```python
from build123d import *

# Parameters (mm, degrees)
F_6_X_6_ANGLE_BAR_EXTRUSION_DEPTH = 63.5
EXTRUSION_FILLETS_R               = 6.35
F_10_CLEARANCE_HOLE_ROUTER_D      = 5.1054
SKETCH7_R                         = 13.49375
F_1_OD_BIT_ACCESS_HOLE_DEPTH      = 219.337526836
TAPPED_HOLE_FOR_10_32_HELICOIL1_D = 5.1054
MOUNTING_SLOTS_REACH              = 226.686


with BuildPart() as part:
    # Sketch1 → 6" x 6" angle bar extrusion (new, symmetric)
    with BuildSketch(Plane(origin=(0, 0, 0), x_dir=(0, 0, -1), z_dir=(1, 0, 0))):
        Polygon((0, 0), (0, 152.4), (-9.525, 152.4), (-9.525, 9.525), (-152.4, 9.525), (-152.4, 0), align=None)
    extrude(amount=F_6_X_6_ANGLE_BAR_EXTRUSION_DEPTH, both=True)

    # extrusion fillets
    extrusion_fillets_edges = [part.edges().sort_by_distance(p)[0] for p in [
        (0, 9.525, 152.4),
        (0, 9.525, 9.525),
        (0, 152.4, 9.525),
    ]]
    fillet(extrusion_fillets_edges, radius=EXTRUSION_FILLETS_R)

    # #10 Clearance Hole - router (through all)
    with Locations(Plane(origin=(0, 9.525, 0), x_dir=(1, 0, 0), z_dir=(0, 1, 0))):
        with Locations((-34.29, -25.4), (34.29, -101.6), (-34.29, -101.6), (34.29, -25.4)):
            Hole(F_10_CLEARANCE_HOLE_ROUTER_D / 2)

    # Sketch7 → 1" OD bit access hole (cut, through all)
    with BuildSketch(Plane(origin=(0, 9.525, 0), x_dir=(1, 0, 0), z_dir=(0, 1, 0))):
        with Locations(Location((-3.4036, -63.5, 0), (0, 0, 270))):
            Circle(SKETCH7_R)
    extrude(amount=-F_1_OD_BIT_ACCESS_HOLE_DEPTH, mode=Mode.SUBTRACT)

    # Tapped Hole for #10-32 Helicoil1 (through all)
    with Locations(Plane(origin=(0, 0, 0), x_dir=(-1, 0, 0), z_dir=(0, -1, 0))):
        with Locations((-53.975, -50.8), (-53.975, -76.2)):
            Hole(TAPPED_HOLE_FOR_10_32_HELICOIL1_D / 2)

    # Sketch14 → mounting slots (cut, up to next)
    with BuildSketch(Plane(origin=(0, 0, 0), x_dir=(-1, 0, 0), z_dir=(0, 0, -1)), mode=Mode.PRIVATE) as mounting_slots_sk1:
        with BuildLine():
            Line((-44.45, 136.525), (-44.45, 130.175))
            ThreePointArc((-44.45, 130.175), (-47.625, 127), (-50.8, 130.175))
            Line((-50.8, 130.175), (-50.8, 136.525))
            ThreePointArc((-50.8, 136.525), (-47.625, 139.7), (-44.45, 136.525))
        make_face()
    mounting_slots_tool1 = extrude(mounting_slots_sk1.sketch, amount=-MOUNTING_SLOTS_REACH, mode=Mode.PRIVATE) & part.part
    # Sketch14 → mounting slots (cut, up to next)
    with BuildSketch(Plane(origin=(0, 0, 0), x_dir=(-1, 0, 0), z_dir=(0, 0, -1)), mode=Mode.PRIVATE) as mounting_slots_sk2:
        with BuildLine():
            Line((-44.45, 85.725), (-44.45, 79.375))
            ThreePointArc((-44.45, 79.375), (-47.625, 76.2), (-50.8, 79.375))
            Line((-50.8, 79.375), (-50.8, 85.725))
            ThreePointArc((-50.8, 85.725), (-47.625, 88.9), (-44.45, 85.725))
        make_face()
    mounting_slots_tool2 = extrude(mounting_slots_sk2.sketch, amount=-MOUNTING_SLOTS_REACH, mode=Mode.PRIVATE) & part.part
    # Sketch14 → mounting slots (cut, up to next)
    with BuildSketch(Plane(origin=(0, 0, 0), x_dir=(-1, 0, 0), z_dir=(0, 0, -1)), mode=Mode.PRIVATE) as mounting_slots_sk3:
        with BuildLine():
            Line((50.8, 85.725), (50.8, 79.375))
            ThreePointArc((50.8, 79.375), (47.625, 76.2), (44.45, 79.375))
            Line((44.45, 79.375), (44.45, 85.725))
            ThreePointArc((44.45, 85.725), (47.625, 88.9), (50.8, 85.725))
        make_face()
    mounting_slots_tool3 = extrude(mounting_slots_sk3.sketch, amount=-MOUNTING_SLOTS_REACH, mode=Mode.PRIVATE) & part.part
    # Sketch14 → mounting slots (cut, up to next)
    with BuildSketch(Plane(origin=(0, 0, 0), x_dir=(-1, 0, 0), z_dir=(0, 0, -1)), mode=Mode.PRIVATE) as mounting_slots_sk4:
        with BuildLine():
            Line((50.8, 136.525), (50.8, 130.175))
            ThreePointArc((50.8, 130.175), (47.625, 127), (44.45, 130.175))
            Line((44.45, 130.175), (44.45, 136.525))
            ThreePointArc((44.45, 136.525), (47.625, 139.7), (50.8, 136.525))
        make_face()
    mounting_slots_tool4 = extrude(mounting_slots_sk4.sketch, amount=-MOUNTING_SLOTS_REACH, mode=Mode.PRIVATE) & part.part
    add(mounting_slots_tool1.solids().sort_by_distance((47.625, 133.35, 0))[0], mode=Mode.SUBTRACT)
    add(mounting_slots_tool2.solids().sort_by_distance((47.625, 82.55, 0))[0], mode=Mode.SUBTRACT)
    add(mounting_slots_tool3.solids().sort_by_distance((-47.625, 82.55, 0))[0], mode=Mode.SUBTRACT)
    add(mounting_slots_tool4.solids().sort_by_distance((-47.625, 133.35, 0))[0], mode=Mode.SUBTRACT)


solid = part.part
```
Here's how the part is built. I have some questions about the finished solid (model axes, mm). A direction names the side the tool comes from. Give positions to 0.01 mm unless a question says otherwise; leave off trailing zeros. Write each loop counter-clockwise with the first axis right and the second up, starting at its lowest first coordinate (ties: lowest second). Pieces come first, ordered by that corner, then holes. Notation, with made-up numbers: (77.25, 43.25) -> (110.25, 43.25) arc R22 ccw to (110.25, 66.25) -> close; hole circle Ø8 at (-37, 41). An arc over 180 degrees is marked (long way). Write each question's results on one line, items separated by ' | '.
Item 1: Suppose I cut it at A-A on z = 25.4. Write out the boundary of the cut face in (x, y) (3 decimals), plus the area to 3 significant figures.
Output:
outline: (-63.5, 0) -> (-36.843, 0) -> (-36.843, 9.525) -> (-63.5, 9.525) -> close; (-31.737, 0) -> (31.737, 0) -> (31.737, 9.525) -> (-31.737, 9.525) -> close; (36.843, 0) -> (63.5, 0) -> (63.5, 9.525) -> (36.843, 9.525) -> close | area: 1,110 mm^2
Item 2: On a 3-axis mill with a long thin cutter (end or side, diameter ignored), from which of +Z, -Z, +X, -X, +Y, -Y can I reach the whole of each face in a straight line? I mean faces 1 (the face through (1, 82, 9.525)), 2 (the face through (36.32, 4.7, 103.15)), 3 (the face through (47.6, 127, 4.7)). Say none if no direction works.
Output:
face 1: +Z, +X, -X, +Y | face 2: +Y, -Y | face 3: +Z, -Z
Item 3: For pin 1 Ø3 at (x, z) = (53.975, 76.2) entering from +Y; pin 2 Ø3 at (x, y) = (-47, 108.5) entering from -Z; pin 3 Ø12 at (x, y) = (-10, 76) entering from +Z (3 decimals); pin 4 Ø6 at (x, z) = (-33.5, 59) entering from +Y (3 decimals), each with a flat end and sliding along its axis, tell me the tip position at first contact or that it passes through.
Output:
pin 1: passes through | pin 2: stops at z = 0 | pin 3: stops at z = 9.525 | pin 4: stops at y = 9.525
Item 4: We'd pull the mould along Z, two halves only. Please class faces 4 (the face through (44.45, 133, 5)), 5 (the face through (56.4, 4.8, 50)), 6 (the face through (0.89, 11.34, 11.43)), 7 (the face through (-35.468, 4.696, 103.865)): pulls with the +Z half, pulls with the -Z half, needs draft (parallel to the pull), parting line crosses it, or undercut.
Output:
face 4: needs draft | face 5: undercut | face 6: pulls with the +Z half | face 7: undercut
Item 5: If I drill on L1, parallel to X at y = 4.5, z = 25.4; L2, parallel to Z at x = 34.29, y = 3.5; L3, parallel to Y at x = -46, z = 36 (3 decimals), over which ranges is the centre line in solid material (lowest first)?
Output:
L1: x = -63.5 to -36.84, -31.74 to 31.74, 36.84 to 63.5 | L2: z = 0 to 22.85, 27.95 to 99.05, 104.15 to 152.39 | L3: y = 0 to 9.525
Item 6: Suppose I cut it at B-B on x = 21.5. Write out the boundary of the cut face in (y, z) (3 decimals), plus the area to 3 significant figures.
Output:
outline: (0, 0) -> (152.4, 0) -> (152.4, 3.175) arc R6.35 ccw to (146.05, 9.525) -> (15.875, 9.525) arc R6.35 cw to (9.525, 15.875) -> (9.525, 146.05) arc R6.35 ccw to (3.175, 152.4) -> (0, 152.4) -> close | area: 2,800 mm^2
Item 7: Suppose I cut it at D-D on x = 34.29. Write out the boundary of the cut face in (y, z) (3 decimals).
Output:
outline: (0, 0) -> (152.4, 0) -> (152.4, 3.175) arc R6.35 ccw to (146.05, 9.525) -> (15.875, 9.525) arc R6.35 cw to (9.525, 15.875) -> (9.525, 22.847) -> (0, 22.847) -> close; (0, 27.953) -> (9.525, 27.953) -> (9.525, 99.047) -> (0, 99.047) -> close; (0, 104.153) -> (9.525, 104.153) -> (9.525, 146.05) arc R6.35 ccw to (3.175, 152.4) -> (0, 152.4) -> close
Item 8: Suppose I cut it at C-C on z = 63.5. Write out the boundary of the cut face in (x, y) (3 decimals).
Output:
outline: (-63.5, 0) -> (-16.897, 0) -> (-16.897, 9.525) -> (-63.5, 9.525) -> close; (10.09, 0) -> (63.5, 0) -> (63.5, 9.525) -> (10.09, 9.525) -> close
